Source: CAD feature listing. Evaluate the final solid. Frame: model axes, mm. A direction names the side the tool comes from. Give positions to 0.01 mm unless a question says otherwise; leave off trailing zeros. Order: outer loops, then holes, each group sorted by start corner. A loop starts at its lowest first (then second) coordinate and runs counter-clockwise, first axis right, second up. Notation, with made-up numbers: (58, -8.75) - (104, -8.75) arc R20 ccw to (104, 10.25) - close; hole circle Ø10 at (83.25, 66). An arc over 180 degrees is marked (long way). One line per item, written item: value. Start each with the question number.
Autodesk Fusion 360 part; units mm, degrees
sketch "Sketch1" plane through (0, 0, 0) normal (0, 0, 1) x (1, 0, 0)
  line L0 (1, 0) -> (51, 0)
  line L1 (52, 1) -> (52, 38)
  line L2 (51, 39) -> (1, 39)
  line L3 (0, 38) -> (0, 1)
  arc A0 (1, 39) -> (0, 38) centre (1, 38) ccw
  arc A1 (52, 38) -> (51, 39) centre (51, 38) ccw
  arc A2 (51, 0) -> (52, 1) centre (51, 1) ccw
  arc A3 (0, 1) -> (1, 0) centre (1, 1) ccw
  line L4 (1.2, 37.8) -> (1.2, 1.2)
  line L5 (1.2, 1.2) -> (50.8, 1.2)
  line L6 (50.8, 1.2) -> (50.8, 37.8)
  line L7 (50.8, 37.8) -> (1.2, 37.8)
  line L8 (49, 3) -> (49, 36)
  line L9 (49, 36) -> (3, 36)
  line L10 (3, 36) -> (3, 3)
  line L11 (3, 3) -> (49, 3)
  point P0 (52, 0)
  point P1 (0, 39)
  dimension "d1" = 52
  dimension "d2" = 39
  dimension "d3" = 1
  dimension "d6" = -1.2
  dimension "d7" = -3
extrude "Extrude1" add sketch "Sketch1" along normal blind 4 contours L0 L1 L2 L3 A0 A1 A2 A3 | L4 L5 L6 L7 | L8 L9 L10 L11
sketch "Sketch2" plane through (0, 0, 4) normal (0, 0, 1) x (-1, 0, 0)
  arc A0 (0, -1) -> (-1, 0) centre (-1, -1) ccw
  line L0 (-1, 0) -> (-51, 0)
  arc A1 (-51, 0) -> (-52, -1) centre (-51, -1) ccw
  line L1 (-52, -1) -> (-52, -38)
  arc A2 (-52, -38) -> (-51, -39) centre (-51, -38) ccw
  line L2 (-51, -39) -> (-1, -39)
  arc A3 (-1, -39) -> (0, -38) centre (-1, -38) ccw
  line L3 (0, -38) -> (0, -1)
sketch "Sketch3" plane through (0, 0, 4) normal (0, 0, 1) x (-1, 0, 0)
extrude "Extrude2" add sketch "Sketch1" against normal blind 3 contours L4 L5 L6 L7
sketch "Sketch4" plane through (0, 0, 4) normal (0, 0, 1) x (-1, 0, 0)
sketch "Sketch5" plane through (0, 0, 4) normal (0, 0, 1) x (-1, 0, 0)
  line L0 (-43.5, -13.25) -> (-36.9, -13.25)
  line L1 (-33.9, -16.25) -> (-33.9, -22.85)
  line L2 (-36.9, -25.85) -> (-43.5, -25.85)
  line L3 (-46.5, -22.85) -> (-46.5, -16.25)
  arc A0 (-43.5, -13.25) -> (-46.5, -16.25) centre (-43.5, -16.25) ccw
  arc A1 (-33.9, -16.25) -> (-36.9, -13.25) centre (-36.9, -16.25) ccw
  arc A2 (-36.9, -25.85) -> (-33.9, -22.85) centre (-36.9, -22.85) ccw
  arc A3 (-46.5, -22.85) -> (-43.5, -25.85) centre (-43.5, -22.85) ccw
  line L4 (-1, 0) -> (-51, 0)
  line L5 (-49, -3) -> (-49, -36)
  line L6 (-29.25, -13.25) -> (-22.65, -13.25)
  arc A4 (-29.25, -13.25) -> (-32.25, -16.25) centre (-29.25, -16.25) ccw
  line L7 (-32.25, -22.85) -> (-32.25, -16.25)
  arc A5 (-32.25, -22.85) -> (-29.25, -25.85) centre (-29.25, -22.85) ccw
  arc A6 (-22.65, -25.85) -> (-19.65, -22.85) centre (-22.65, -22.85) ccw
  line L8 (-22.65, -25.85) -> (-29.25, -25.85)
  line L9 (-19.65, -16.25) -> (-19.65, -22.85)
  arc A7 (-19.65, -16.25) -> (-22.65, -13.25) centre (-22.65, -16.25) ccw
  line L10 (-15, -13.25) -> (-8.4, -13.25)
  arc A8 (-15, -13.25) -> (-18, -16.25) centre (-15, -16.25) ccw
  line L11 (-18, -22.85) -> (-18, -16.25)
  arc A9 (-18, -22.85) -> (-15, -25.85) centre (-15, -22.85) ccw
  arc A10 (-8.4, -25.85) -> (-5.4, -22.85) centre (-8.4, -22.85) ccw
  line L12 (-8.4, -25.85) -> (-15, -25.85)
  line L13 (-5.4, -16.25) -> (-5.4, -22.85)
  arc A11 (-5.4, -16.25) -> (-8.4, -13.25) centre (-8.4, -16.25) ccw
  point P0 (-46.5, -13.25)
  point P1 (-33.9, -13.25)
  point P2 (-46.5, -25.85)
  dimension "d10" = 12.6
  dimension "d11" = 12.6
  dimension "d12" = 3
  dimension "d13" = 13.25
  dimension "d14" = 2.5
  dimension "d17" = 14.25
  dimension "d18" = 0
extrude "Extrude3" cut sketch "Sketch5" against normal blind 8
1. Section B-B on x = 11.5. Return the cut outline in (y, z), then the cut area to 3 significant figures.
2. Section A-A on y = 17. Return the cut outline in (x, z), then the cut area to 3 significant figures.
3. Draft query along Y for faces 1 (the flat face through (26, 12, 0)), 2 (the flat face through (26, 1.2, -1)), 3 (the flat face through (24, 1, 0)). Return one class per face: pulls with the +Y half, pulls with the -Y half, needs draft (parallel to the pull), parting line crosses it, or undercut.
4. Section D-D on z = 1.5. Count the separate pieces of the cut face and the enclosed holes in it, then the cut area to 3 significant figures.
5. Section C-C on z = -1.75. Return the cut outline in (x, y).
6. Contact query for flat-ended pins moving along their axis: pin 1 Ø0.9 at (x, z) = (36, -2) entering from +Y; pin 2 Ø1.5 at (y, z) = (15, -1) entering from +X; pin 3 Ø1.5 at (x, y) = (20, 11) entering from -Z. Output: stop coordinate, or through.
7. Set-up query: faces 4 (the flat face through (3, 20, -1)), 5 (the flat face through (12, 25.85, 2)), 6 (the cylindrical face through (51.699, 38.715, 1.972)). Return all of +Z, -Z, +X, -X, +Y, -Y with unobstructed straight access to the full face (end or side cutting, diameter ignored); none if empty.
8. Ray query, L1, parallel to X at y = 28, z = -0.5; L2, parallel to X at y = 23, z = 2.75; L3, parallel to X at y = 24, z = 0.5. Return the intervals inside material, ascending.
Data:
1. outline: (0, 0) - (1.2, 0) - (1.2, -3) - (3, -3) - (3, 0) - (13.25, 0) - (13.25, 4) - (0, 4) - close; (25.85, 0) - (36, 0) - (36, -3) - (37.8, -3) - (37.8, 0) - (39, 0) - (39, 4) - (25.85, 4) - close
1. area: 116 mm2
2. outline: (0, 0) - (1.2, 0) - (1.2, -3) - (3, -3) - (3, 0) - (5.4, 0) - (5.4, 4) - (0, 4) - close; (18, 0) - (19.65, 0) - (19.65, 4) - (18, 4) - close; (32.25, 0) - (33.9, 0) - (33.9, 4) - (32.25, 4) - close; (46.5, 0) - (49, 0) - (49, -3) - (50.8, -3) - (50.8, 0) - (52, 0) - (52, 4) - (46.5, 4) - close
2. area: 67.6 mm2
3. face 1: undercut
3. face 2: pulls with the -Y half
3. face 3: needs draft
4. separate pieces: 1
4. enclosed holes: 3
4. area: 1,570 mm2
5. outline: (1.2, 1.2) - (50.8, 1.2) - (50.8, 37.8) - (1.2, 37.8) - close; hole (3, 3) - (49, 3) - (49, 36) - (3, 36) - close
6. pin 1: stops at y = 37.8
6. pin 2: stops at x = 50.8
6. pin 3: stops at z = 0
7. face 4: -Z
7. face 5: +Z, -Z
7. face 6: +Z, -Z, +X, +Y
8. L1: x = 1.2 to 3, 49 to 50.8
8. L2: x = 0 to 5.4, 18 to 19.65, 32.25 to 33.9, 46.5 to 52
8. L3: x = 0 to 5.63, 17.77 to 19.88, 32.02 to 34.13, 46.27 to 52
